```python
from build123d import *

# Parameters (mm, degrees)
BOSS_EXTRUDE1_DEPTH = 6
SKETCH2_W           = 0.4
SKETCH2_H           = 0.4
BOSS_EXTRUDE2_DEPTH = 5.5


with BuildPart() as part:
    # Sketch1 → Boss-Extrude1 (new body)
    with BuildSketch(Plane.XY):
        Polygon((-5, 7), (-5, -4), (5, -4), (5, 7), (9.75, 7), (9.75, -7), (-9.75, -7), (-9.75, 7), align=None)
    extrude(amount=BOSS_EXTRUDE1_DEPTH)

    # Sketch2 → Boss-Extrude2 (add)
    with BuildSketch(Plane.XZ.offset(7)):
        with Locations((-7.45, 3.874333009)):
            Rectangle(SKETCH2_W, SKETCH2_H)
        with Locations((7.45, 3.874333009)):
            Rectangle(SKETCH2_W, SKETCH2_H)
        with Locations((7.45, 0.934333009)):
            Rectangle(SKETCH2_W, SKETCH2_H)
        with Locations((-7.45, 0.934333009)):
            Rectangle(SKETCH2_W, SKETCH2_H)
    extrude(amount=BOSS_EXTRUDE2_DEPTH)


solid = part.part
```
Can you work these out from the model? Positions are in its coordinate system, mm. A direction names the side the tool comes from. Round coordinates to 2 decimals unless told otherwise and drop trailing zeros. Loops run counter-clockwise (first coordinate to the right, second up) from the corner with the lowest first, then second, coordinate; pieces in that order, holes last.
Item 1: Which directions (+Z, -Z, +X, -X, +Y, -Y) give clear straight access to the entire face, cutting with the end or side of a thin tool? Please do faces 1 (the flat face through (-5, 2, 3)), 2 (the flat face through (0, -5, 6)).
Item 2: If we mould it in two halves opening along X, with no side actions, what happens to faces 3 (the flat face through (5, 1, 3)), 4 (the flat face through (-7, 7, 3)), 5 (the flat face through (-9.75, 0, 3))? For each: +X half, -X half, draft (parallel to the pull), parting line (faces both ways), or undercut.
Item 3: Suppose I cut it at A-A, the plane y = -1.5. Write out the boundary of the cut face in (x, z), then the cut area to 3 significant figures.
Item 4: Suppose I cut it at B-B, the plane y = -10. Write out the boundary of the cut face in (x, z), then the cut area to 3 significant figures.
Item 5: Suppose I cut it at C-C, the plane z = 4.45. Write out the boundary of the cut face in (x, y).
Item 6: Suppose I cut it at D-D, the plane x = -1.25. Write out the boundary of the cut face in (y, z), then the cut area to 3 significant figures.
Item 7: Please list where these lines run through material, in increasing order: L1, parallel to X at y = -10.5, z = 0.9; L2, parallel to X at y = -2, z = 3.25; L3, parallel to Y at x = -8.5, z = 0.55.
Reported:
1. face 1: +Z, -Z, +Y
1. face 2: +Z, +X, -X, +Y, -Y
2. face 3: undercut
2. face 4: draft
2. face 5: -X half
3. outline: (-9.75, 0) - (-5, 0) - (-5, 6) - (-9.75, 6) - close; (5, 0) - (9.75, 0) - (9.75, 6) - (5, 6) - close
3. area: 57.0 mm2
4. outline: (-7.65, 0.73) - (-7.25, 0.73) - (-7.25, 1.13) - (-7.65, 1.13) - close; (-7.65, 3.67) - (-7.25, 3.67) - (-7.25, 4.07) - (-7.65, 4.07) - close; (7.25, 0.73) - (7.65, 0.73) - (7.65, 1.13) - (7.25, 1.13) - close; (7.25, 3.67) - (7.65, 3.67) - (7.65, 4.07) - (7.25, 4.07) - close
4. area: 0.640 mm2
5. outline: (-9.75, -7) - (9.75, -7) - (9.75, 7) - (5, 7) - (5, -4) - (-5, -4) - (-5, 7) - (-9.75, 7) - close
6. outline: (-7, 0) - (-4, 0) - (-4, 6) - (-7, 6) - close
6. area: 18.0 mm2
7. L1: x = -7.65 to -7.25, 7.25 to 7.65
7. L2: x = -9.75 to -5, 5 to 9.75
7. L3: y = -7 to 7
